Can you work these out from the model? Positions are in its coordinate system, mm. Face numbers are marked on the shaded views. Round coordinates to 2 decimals unless told otherwise and drop trailing zeros. Order: outer loops, then holes, each group sorted by start corner. A loop starts at its lowest first (then second) coordinate and runs counter-clockwise, first axis right, second up. Notation, with made-up numbers: M 89.5,1 L 108.5,1 A16 cw 108.5,30 Z; hole C 57,10.25 d10. An arc over 180 degrees is marked long. Answer as a JSON object with one key per item and string values. Group by question number.
Autodesk Inventor part; units mm, degrees
ref_plane "YZ Plane" through (0, 0, 0) normal (1, 0, 0) x (0, 1, 0)
ref_plane "XZ Plane" through (0, 0, 0) normal (0, 1, 0) x (-1, 0, 0)
ref_plane "XY Plane" through (0, 0, 0) normal (0, 0, 1) x (1, 0, 0)
sketch "Sketch1" plane through (0, 0, 0) normal (0, 1, 0) x (-1, 0, 0)
  circle A0 centre (-0.0502, 38.3312) radius 4.925
  line L0 (-0.0502, 38.3312) -> (0, 0)
  circle A1 centre (38.3312, 0.0502) radius 4.925
  line L1 (38.3312, 0.0502) -> (0, 0)
  circle A2 centre (38.3312, 0.0502) radius 5
  circle A3 centre (-0.0502, 38.3312) radius 5
  circle A4 centre (-0.0502, 38.3312) radius 7.5
  circle A5 centre (38.3312, 0.0502) radius 7.5
  line L2 (38.3312, 0.0502) -> (-0.0502, 38.3312)
  line L3 (21.6405, 21.6907) -> (16.6405, 21.6907)
  line L4 (16.6405, 21.6907) -> (16.6405, 16.6907)
  line L5 (16.6405, 16.6907) -> (21.6405, 16.6907)
  line L6 (21.6405, 16.6907) -> (21.6405, 21.6907)
  line L7 (21.6405, 21.6907) -> (16.6405, 16.6907) construction
  line L8 (16.6405, 21.6907) -> (21.6405, 16.6907) construction
  line L9 (21.6405, 21.6907) -> (2.4716, 40.8596)
  line L10 (21.6405, 21.6907) -> (37.3312, 6)
  line L11 (16.6405, 16.6907) -> (-2.5284, 35.8596)
  line L12 (16.6405, 16.6907) -> (32.3312, 1)
  point P0 (0, 0)
  point P1 (0, 0)
  point P2 (19.1405, 19.1907)
  point P3 (36.1157, 7.2155)
  point P4 (7.1385, 36.1927)
  point P5 (2.1653, 31.1659)
  point P6 (31.1425, 2.1887)
  dimension "d0" = 10
  dimension "d1" = 10
  dimension "d2" = 15
  dimension "d3" = 15
  dimension "d4" = 5
  dimension "d5" = 5
extrude "Extrusion1" add sketch "Sketch1" along normal blind 5 contours L9 A4 L2 A3 | A3 L0 A4 L9 | L2 A4 L11 A3 | A3 L11 A4 L0 | L9 L3 L4 L2 A4 | L2 L4 L11 A4 | L6 L2 L4 L3 | L10 A5 L2 L6 | L2 L6 L5 L4 | L2 A5 L12 L5 L6 | A5 L1 A2 L2 | A5 L2 A2 L1
properties part number "Pillar_corner_v2"
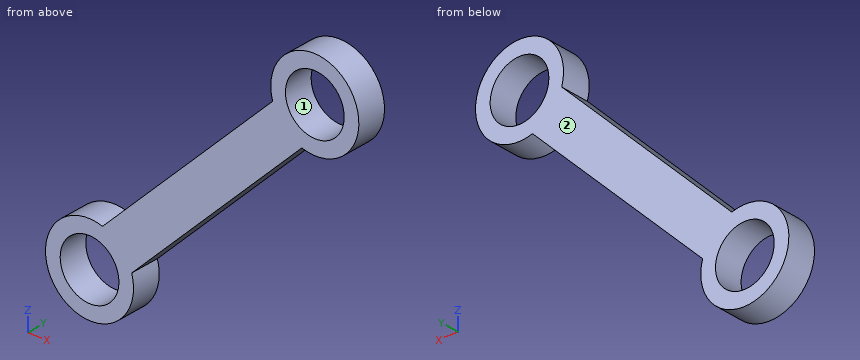
Item 1: Suppose I cut it at D-D, the plane z = 24.5. Write out the boundary of the cut face in (x, y), and give its area (3 significant figures).
Item 2: I need wall thicknesses on line 1 (X direction, y = 1.25, z = 0.5); line 2 (X direction, y = 1.95, z = 38); line 3 (Z direction, x = -41, y = 2.5). Which ranges of each line are inside material? Lowest first, please.
Item 3: I'm going to push flat-ended pins straight in: pin 1 Ø11.5 at (x, z) = (0.05, 38.33) entering from +Y; pin 2 Ø2 at (y, z) = (1.5, 15) entering from +X; pin 3 Ø3 at (x, y) = (-0.5, 4) entering from -Z. Where does each tip first touch, or does it pass through?
Item 4: Suppose I cut it at B-B, the plane x = -41.5. Write out the boundary of the cut face in (y, z), and give its area (3 significant figures).
Item 5: Suppose I cut it at A-A, the plane z = 1.5. Write out the boundary of the cut face in (x, y), and give its area (3 significant figures).
Item 6: If we mould it in two halves opening along Z, with no side actions, what happens to the marked faces 1 and 2? For each: +Z half, -Z half, draft (parallel to the pull), parting line (faces both ways), or undercut.
Item 7: Suppose I cut it at C-C, the plane y = 1.6. Write out the boundary of the cut face in (x, z), and give its area (3 significant figures).
Computed:
{
 "1": {"outline": "M -18.83,0 L -8.83,0 L -8.83,5 L -18.83,5 Z", "area": "50.0 mm^2"},
 "2": {"line 1": "x = -45.82 to -43.31, -33.35 to -30.84", "line 2": "x = -7.44 to -4.94, 5.04 to 7.54", "line 3": "z = -6.96 to -4.18, 4.28 to 7.06"},
 "3": {"pin 1": "stops at y = 5", "pin 2": "stops at x = -17.33", "pin 3": "stops at z = 30.83"},
 "4": {"outline": "M 0,-6.75 L 5,-6.75 L 5,-3.82 L 0,-3.82 Z; M 0,3.92 L 5,3.92 L 5,6.85 L 0,6.85 Z", "area": "29.3 mm^2"},
 "5": {"outline": "M -45.69,0 L -43.12,0 L -43.12,5 L -45.69,5 Z; M -33.55,0 L -30.97,0 L -30.97,5 L -33.55,5 Z", "area": "25.7 mm^2"},
 "6": {"face 1": "undercut", "face 2": "draft"},
 "7": {"outline": "M -36.12,7.22 A7.5 ccw long -31.14,2.19 L -2.17,31.17 A7.5 ccw long -7.14,36.19 Z; hole C -38.33,0.05 d10; hole C 0.05,38.33 d10", "area": "478 mm^2"}
}
